Build history of the part. All positions in model axes, mm. A direction names the side the tool comes from. Give positions to 0.01 mm unless a question says otherwise; leave off trailing zeros. Order: outer loops, then holes, each group sorted by start corner. A loop starts at its lowest first (then second) coordinate and runs counter-clockwise, first axis right, second up. Notation, with made-up numbers: (72.5, -35.5) - (88.5, -35.5) arc R25 ccw to (88.5, -17.5) - close; hole circle Ø5 at (-35.5, -2). An arc over 180 degrees is marked (long way). Use a Markdown table: item, result.
from build123d import *

# Parameters (mm, degrees)
F0_W          = 76.034322
F0_H          = 32.407026
F1_DEPTH      = 25
F1_DEPTH_BACK = 25
F2_R          = 18.431692
F2_R_2        = 13.728348
F3_DEPTH      = 11.3
F3_FACE_R     = 13.728348
F4_DEPTH      = 32.407027


with BuildPart() as f1:
    # F0 (on Top) → F1 (new body, two sides)
    with BuildSketch(Plane.XY) as f1_sk:
        Rectangle(F0_W, F0_H)
    extrude(amount=F1_DEPTH)
    extrude(f1_sk.sketch, amount=-F1_DEPTH_BACK)

    # F2 (on face) → F3 (join)
    with BuildSketch(Plane.XZ.offset(16.203513)):
        Circle(F2_R)
        Circle(F2_R_2, mode=Mode.SUBTRACT)
    extrude(amount=F3_DEPTH)

    # F3_face (on face) → F4 (cut, through all)
    with BuildSketch(Plane.XZ.offset(16.203513)):
        Circle(F3_FACE_R)
    extrude(amount=-F4_DEPTH, mode=Mode.SUBTRACT)


solid = f1.part
1) Slice it at A-A (z = 0). Write the cut outline in (x, y).
Computed:
| item | result |
|---|---|
| outline | (-38.02, -16.2) - (-18.43, -16.2) - (-18.43, -27.5) - (-13.73, -27.5) - (-13.73, 16.2) - (-38.02, 16.2) - close; (13.73, -27.5) - (18.43, -27.5) - (18.43, -16.2) - (38.02, -16.2) - (38.02, 16.2) - (13.73, 16.2) - close |
2) Slice it at D-D (x = -16.5). Write the cut outline in (y, z).
Computed:
| item | result |
|---|---|
| outline | (-27.5, -8.21) - (-16.2, -8.21) - (-16.2, -25) - (16.2, -25) - (16.2, 25) - (-16.2, 25) - (-16.2, 8.21) - (-27.5, 8.21) - close |
3) Slice it at B-B (x = 0). Write the cut outline in (y, z), and give its area (3 significant figures).
Computed:
| item | result |
|---|---|
| outline | (-27.5, -18.43) - (-16.2, -18.43) - (-16.2, -25) - (16.2, -25) - (16.2, -13.73) - (-27.5, -13.73) - close; (-27.5, 13.73) - (16.2, 13.73) - (16.2, 25) - (-16.2, 25) - (-16.2, 18.43) - (-27.5, 18.43) - close |
| area | 837 mm² |
4) Wall check: line 1 (Z direction, x = 0, y = -22.5); line 2 (Y direction, x = -28.5, z = 1.5); line 3 (Z direction, x = 0, y = -8). Give the ranges that are in metal, low to high. Write a range as from..to.
Computed:
| item | result |
|---|---|
| line 1 | z = -18.43..-13.73, 13.73..18.43 |
| line 2 | y = -16.2..16.2 |
| line 3 | z = -25..-13.73, 13.73..25 |
5) Slice it at C-C (y = -14). Write the cut outline in (x, z).
Computed:
| item | result |
|---|---|
| outline | (-38.02, -25) - (38.02, -25) - (38.02, 25) - (-38.02, 25) - close; hole circle Ø27.46 at (0, 0) |
6) Tool access for faces 1 (the flat face through (-9, -16.204, 17)), 2 (the flat face through (-1, 0, 25)): list every direction of +Z, -Z, +X, -X, +Y, -Y with a clear straight run to the whole face (end or side of a thin tool).
Computed:
| item | result |
|---|---|
| face 1 | -Y |
| face 2 | +Z, +X, -X, +Y, -Y |
